Verification items for the finished model (mm, model axes). A direction names the side the tool comes from. Round coordinates to 2 decimals unless told otherwise and drop trailing zeros. Write each loop counter-clockwise with the first axis right and the second up, starting at its lowest first coordinate (ties: lowest second). Pieces come first, ordered by that corner, then holes. Notation, with made-up numbers: M -2,88.5 L 32,88.5 A26 ccw 32,111.5 Z; hole C 63,41.5 d1. An arc over 180 degrees is marked long. One line per question, with ' | ' between items.
from build123d import *

# Parameters (mm, degrees)
F0_R          = 2.625
F1_DEPTH      = 70
F2_W          = 17.5
F2_H          = 25
F3_DEPTH      = 16
F5_W          = 14
F5_H          = 10
F6_DEPTH      = 9
F6_DEPTH_BACK = 5.001
F7_R          = 4.99999
F8_ANGLE      = 180
F9_ANGLE      = 180


# Not quite as in the source:
# - a fillet or chamfer is up to 0.001 mm smaller than in the source, because OpenCascade refuses the exact size


with BuildPart() as f1:
    # F0 (on Right) → F1 (new body)
    with BuildSketch(Plane.YZ):
        with BuildLine():
            Line((-5, 5), (-20.3439258039, 5))
            Line((-20.3439258039, 5), (-75, 5))
            ThreePointArc((-75, 5), (-79.3301270189, -2.5), (-70.6698729811, -2.5))
            ThreePointArc((-70.6698729811, -2.5), (-68.8397459622, -0.6698729811), (-66.3397459622, 0))
            Line((-66.3397459622, 0), (0, 0))
            Line((0, 0), (0, 5))
            Line((0, 5), (0, 25))
            Line((0, 25), (-15, 25))
            Line((-15, 25), (-15, 20))
            Line((-15, 20), (-5, 20))
            Line((-5, 20), (-5, 5))
        make_face()
        with Locations((-75, 0)):
            Circle(F0_R, mode=Mode.SUBTRACT)
    extrude(amount=F1_DEPTH)

    # F2 (on Front) → F3 (cut)
    with BuildSketch(Plane.XZ):
        with Locations((8.75, 12.5)):
            Rectangle(F2_W, F2_H)
        with Locations((61.25, 12.5)):
            Rectangle(F2_W, F2_H)
    extrude(amount=F3_DEPTH, mode=Mode.SUBTRACT)

    # F5 (on offset) → F6 (cut, two sides)
    with BuildSketch(Plane.XZ.offset(75)) as f6_sk:
        with Locations((7, 0)):
            Rectangle(F5_W, F5_H)
        with Locations((35, 0)):
            Rectangle(F5_W, F5_H)
        with Locations((63, 0)):
            Rectangle(F5_W, F5_H)
    extrude(amount=-F6_DEPTH, mode=Mode.SUBTRACT)
    extrude(f6_sk.sketch, amount=F6_DEPTH_BACK, mode=Mode.SUBTRACT)

    # F7 (radius 5 in the source; OpenCascade refuses exactly that, so slightly less here)
    f7_edges = [f1.edges().sort_by_distance(p)[0] for p in [
        (35, -15, 25),
    ]]
    fillet(f7_edges, radius=F7_R)


with BuildPart() as f1_1:
    # F8: moved
    add(f1.part.rotate(Axis((56, -75, 0), (-1, 0, 0)), F8_ANGLE))


with BuildPart() as f1_2:
    # F9: moved
    add(f1_1.part.rotate(Axis((70, -109, 0), (0, -1, 0)), F9_ANGLE))


solid = f1_2.part
1. Section check C-C, the plane z = 1.25. Record the cut outline in (x, y), then the cut area to 3 significant figures.
Results:
outline: M 70,-134 L 87.5,-134 L 87.5,-150 L 122.5,-150 L 122.5,-134 L 140,-134 L 140,-84 L 126,-84 L 126,-77.31 L 112,-77.31 L 112,-84 L 98,-84 L 98,-77.31 L 84,-77.31 L 84,-84 L 70,-84 Z; M 84,-72.69 L 98,-72.69 L 98,-70.16 L 84,-70.16 Z; M 112,-72.69 L 126,-72.69 L 126,-70.16 L 112,-70.16 Z | area: 4,320 mm2
2. Tool access check on faces 4 (the face through (87.5, -146, 12)), 5 (the face through (105, -140, 20)), 6 (the face through (131, -134, 3)). Record the directions out of +Z, -Z, +X, -X, +Y, -Y that give a thin tool (end or side, any length) a straight path to the whole face; none if there is none.
Results:
face 4: +Z, -Z, -X, -Y | face 5: +X, -X, +Y | face 6: +Z, -Z, +X, -Y
3. Go/stop test with flat-tipped pins: P1, Ø2.5, axis at x = 81, z = 2.5, coming from the -Y side; P2, Ø13, axis at y = -145, z = 18.5, coming from the +X side; P3, Ø6, axis at y = -75, z = 0, coming from the +X side; P4, Ø8, axis at y = -128, z = 20.5, coming from the +X side. Record where each tip stops, or that it passes through.
Results:
P1: stops at y = -134 | P2: stops at x = 122.5 | P3: stops at x = 126 | P4: passes through
4. Section check A-A, the plane y = -142.5. Record the cut outline in (x, z), then the cut area to 3 significant figures.
Results:
outline: M 87.5,0 L 122.5,0 L 122.5,5 L 87.5,5 Z; M 87.5,20 L 122.5,20 L 122.5,25 L 87.5,25 Z | area: 350 mm2
5. Thickness scan on line 1 (Z direction, x = 100, y = -142); line 2 (Y direction, x = 91.5, z = 9.5); line 3 (Z direction, x = 97.5, y = -102.5). Record the ranges inside material, lowest first.
Results:
line 1: z = 0 to 5, 20 to 25 | line 2: y = -150 to -145 | line 3: z = 0 to 5
6. Mould release check, pull along Z, two halves, no side actions. Record for faces 1 (the face through (105, -116, 0)), 2 (the face through (79, -134, 3)), 3 (the face through (105, -145, 13)): pulls with the +Z half, pulls with the -Z half, needs draft (parallel to the pull), parting line crosses it, or undercut.
Results:
face 1: pulls with the -Z half | face 2: needs draft | face 3: undercut
